from build123d import *

# Parameters (mm, degrees)
F0_R      = 1.5
F0_R_2    = 5.3160889555
F1_DEPTH  = 4
F2_SIZE   = 5
F3_W      = 25
F3_H      = 4
F4_DEPTH  = 15
F5_W      = 25
F5_H      = 15
F6_DEPTH  = 4
F7_R      = 1.65
F8_DEPTH  = 25
F9_R      = 1.65
F10_DEPTH = 25
F11_W     = 4
F11_H     = 18.4155227914
F11_H_2   = 18
F12_DEPTH = 15
F14_DEPTH = 28.2
F15_R     = 3.349705052
F16_DEPTH = 25
F17_SIZE  = 5


with BuildPart() as f1:
    # F0 (on Top) → F1 (new body)
    with BuildSketch(Plane.XY):
        with BuildLine():
            Line((12.5, -10.5), (12.5, 10.5))
            Line((12.5, 10.5), (-12.5, 10.5))
            Line((-12.5, 10.5), (-12.5, -10.5))
            ThreePointArc((-12.5, -10.5), (-11.9142135624, -11.9142135624), (-10.5, -12.5))
            Line((-10.5, -12.5), (10.5, -12.5))
            ThreePointArc((10.5, -12.5), (11.9142135624, -11.9142135624), (12.5, -10.5))
        make_face()
        with Locations((-5.6568542495, -5.6568542495)):
            Circle(F0_R, mode=Mode.SUBTRACT)
        with Locations((5.6568542495, -5.6568542495)):
            Circle(F0_R, mode=Mode.SUBTRACT)
        with Locations((-5.6568542495, 5.6568542495)):
            Circle(F0_R, mode=Mode.SUBTRACT)
        Circle(F0_R_2, mode=Mode.SUBTRACT)
        with Locations((5.6568542495, 5.6568542495)):
            Circle(F0_R, mode=Mode.SUBTRACT)
        with BuildLine():
            Line((12.5, -16.5), (12.5, -10.5))
            ThreePointArc((12.5, -10.5), (11.9142135624, -11.9142135624), (10.5, -12.5))
            Line((10.5, -12.5), (-10.5, -12.5))
            ThreePointArc((-10.5, -12.5), (-11.9142135624, -11.9142135624), (-12.5, -10.5))
            Line((-12.5, -10.5), (-12.5, -16.5))
            Line((-12.5, -16.5), (-10.5, -16.5))
            Line((-10.5, -16.5), (10.5, -16.5))
            Line((10.5, -16.5), (12.5, -16.5))
        make_face()
    extrude(amount=F1_DEPTH)

    # F2
    f2_edges = [f1.edges().sort_by_distance(p)[0] for p in [
        (12.5, 10.5, 2),
        (-12.5, 10.5, 2),
    ]]
    chamfer(f2_edges, length=F2_SIZE)

    # F3 (on face) → F4 (join)
    with BuildSketch(Plane.XY.offset(4)):
        with Locations((0, -14.5)):
            Rectangle(F3_W, F3_H)
    extrude(amount=F4_DEPTH)

    # F5 (on face) → F6 (join)
    with BuildSketch(Plane(origin=(0, 0, 0), x_dir=(1, 0, 0), z_dir=(0, 0, -1))):
        with Locations((0, 24)):
            Rectangle(F5_W, F5_H)
    extrude(amount=-F6_DEPTH)

    # F7 (on face) → F8 (cut)
    with BuildSketch(Plane.XZ.offset(16.5)):
        with Locations((-7.1815280244, 11.5)):
            Circle(F7_R)
        with Locations((7.0133642294, 11.5)):
            Circle(F7_R)
    extrude(amount=-F8_DEPTH, mode=Mode.SUBTRACT)

    # F9 (on face) → F10 (cut)
    with BuildSketch(Plane.XY.offset(4)):
        with Locations((0, -24)):
            Circle(F9_R)
    extrude(amount=-F10_DEPTH, mode=Mode.SUBTRACT)

    # F11 (on face) → F12 (join, through all)
    with BuildSketch(Plane.XY.offset(4)):
        with Locations((-10.5, -3.7077613957)):
            Rectangle(F11_W, F11_H)
        with Locations((10.5, -3.5)):
            Rectangle(F11_W, F11_H_2)
    extrude(amount=F12_DEPTH)

    # F13 (on face) → F14 (cut)
    with BuildSketch(Plane(origin=(-12.5, 0, 0), x_dir=(0, -1, 0), z_dir=(-1, 0, 0))):
        Polygon((-5.5, 4), (12.5, 19), (-5.5, 19), align=None)
    extrude(amount=-F14_DEPTH, mode=Mode.SUBTRACT)

    # F15 (on face) → F16 (cut)
    with BuildSketch(Plane(origin=(0, -12.5, 0), x_dir=(-1, 0, 0), z_dir=(0, 1, 0))):
        with Locations((-7.0133642294, 11.5)):
            Circle(F15_R)
        with Locations((7.1815280244, 11.5)):
            Circle(F15_R)
    extrude(amount=F16_DEPTH, mode=Mode.SUBTRACT)

    # F17
    f17_edges = [f1.edges().sort_by_distance(p)[0] for p in [
        (-12.5, -31.5, 2),
        (12.5, -31.5, 2),
    ]]
    chamfer(f17_edges, length=F17_SIZE)


solid = f1.part
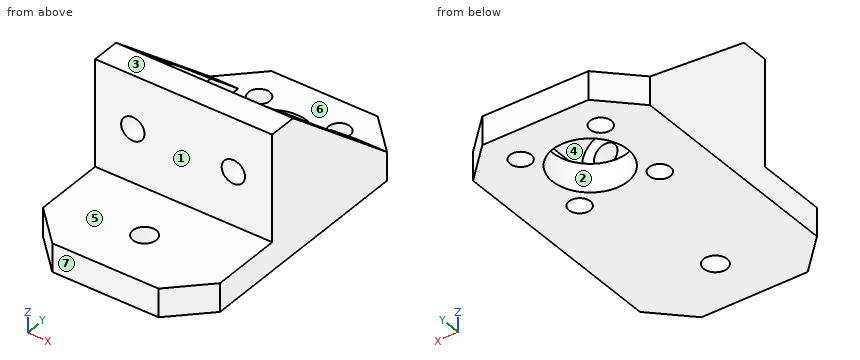
Verification items for the finished model (mm, model axes). Face numbers are marked on the shaded views. A direction names the side the tool comes from. Coordinates: 2 decimals unless noted, no trailing zeros. Loops run counter-clockwise (first coordinate to the right, second up) from the corner with the lowest first, then second, coordinate; pieces in that order, holes last. Notation, with made-up numbers: (77.25, 80.5) -> (102.25, 80.5) arc R20 cw to (102.25, 103.5) -> close; hole circle Ø5 at (6.5, 16). An arc over 180 degrees is marked (long way). Answer as a JSON object with one key per item and string values. Group by question number.
Item 1: Mould release check, pull along Y, two halves, no side actions. Record for the marked faces 1, 2 and 3: +Y half, -Y half, draft (parallel to the pull), parting line (faces both ways), or undercut.
Item 2: Sectioned sample at C-C on y = -24. Record the boundary of the cut face in (x, z), plus the area to 3 significant figures.
Item 3: Sectioned sample at D-D on z = 2. Record the boundary of the cut face in (x, y).
Item 4: Tool access check on the marked faces 4, 5, 6 and 7. Record the directions out of +Z, -Z, +X, -X, +Y, -Y that give a thin tool (end or side, any length) a straight path to the whole face; none if there is none.
Item 5: Sectioned sample at A-A on z = 11.5. Record the boundary of the cut face in (x, y), plus the area to 3 significant figures.
Item 6: Sectioned sample at B-B on x = 0. Record the boundary of the cut face in (y, z), plus the area to 3 significant figures.
Item 7: Depth check by flat-ended pin: pin 1 (3.5 mm diameter, centred on x = -5.66, y = 5.66, fed in from +Z); pin 2 (3 mm diameter, centred on x = -9.5, z = 11, fed in from -Y); pin 3 (4 mm diameter, centred on x = 7.01, z = 11.5, fed in from +Y). Enter the tip coordinate at first touch or a pass-through.
Item 8: Scan lines: probe 1 along Y at (x, z) = (0, 2.75); probe 2 along X at (y, z) = (-11, 15.75); probe 3 along Z at (x, y) = (-10.75, 5.5). Record each from-to range of solid material in increasing order.
Evaluation:
{
 "1": {"face 1": "-Y half", "face 2": "undercut", "face 3": "draft"},
 "2": {"outline": "(-12.5, 0) -> (-1.65, 0) -> (-1.65, 4) -> (-12.5, 4) -> close; (1.65, 0) -> (12.5, 0) -> (12.5, 4) -> (1.65, 4) -> close", "area": "86.8 mm²"},
 "3": {"outline": "(-12.5, -26.5) -> (-7.5, -31.5) -> (7.5, -31.5) -> (12.5, -26.5) -> (12.5, 5.5) -> (7.5, 10.5) -> (-7.5, 10.5) -> (-12.5, 5.5) -> close; hole circle Ø3 at (-5.66, -5.66); hole circle Ø3 at (-5.66, 5.66); hole circle Ø10.63 at (0, 0); hole circle Ø3.3 at (0, -24); hole circle Ø3 at (5.66, -5.66); hole circle Ø3 at (5.66, 5.66)"},
 "4": {"face 4": "+Y", "face 5": "+Z, +X, -X, -Y", "face 6": "+Z, +Y", "face 7": "+Z, -Z, +X, -X, -Y"},
 "5": {"outline": "(-12.5, -16.5) -> (-8.83, -16.5) -> (-8.83, -12.92) -> (-8.5, -12.92) -> (-8.5, -12.5) -> (-10.53, -12.5) -> (-10.53, -3.5) -> (-12.5, -3.5) -> close; (-5.53, -16.5) -> (5.36, -16.5) -> (5.36, -12.5) -> (-5.53, -12.5) -> close; (8.66, -16.5) -> (12.5, -16.5) -> (12.5, -3.5) -> (10.36, -3.5) -> (10.36, -12.5) -> (8.66, -12.5) -> close", "area": "111 mm²"},
 "6": {"outline": "(-31.5, 0) -> (-25.65, 0) -> (-25.65, 4) -> (-31.5, 4) -> close; (-22.35, 0) -> (-5.32, 0) -> (-5.32, 4) -> (-12.5, 4) -> (-12.5, 19) -> (-16.5, 19) -> (-16.5, 4) -> (-22.35, 4) -> close; (5.32, 0) -> (10.5, 0) -> (10.5, 4) -> (5.32, 4) -> close", "area": "172 mm²"},
 "7": {"pin 1": "stops at z = 4", "pin 2": "stops at y = -16.5", "pin 3": "stops at y = -12.5"},
 "8": {"probe 1": "y = -31.5 to -25.65, -22.35 to -5.32, 5.32 to 10.5", "probe 2": "x = -12.5 to -8.5, 8.5 to 12.5", "probe 3": "z = 0 to 4"}
}
